Check sheet for the modelled part. Datum: model origin and axes. Units: mm. A direction names the side the tool comes from. Give positions to 0.01 mm unless a question says otherwise; leave off trailing zeros. Order: outer loops, then holes, each group sorted by start corner. A loop starts at its lowest first (then second) coordinate and runs counter-clockwise, first axis right, second up. Notation, with made-up numbers: (34.25, 2.5) -> (57.25, 2.5) arc R30 cw to (57.25, 27.5) -> close; hole circle Ø1 at (4.5, 58). An arc over 180 degrees is marked (long way). One line per question, with ' | ' between items.
```python
from build123d import *

# Parameters (mm, degrees)
BOSS_EXTRUDE1_DEPTH    = 6
SKETCH2_W              = 98
SKETCH2_H              = 80.5
CUT_EXTRUDE1_DEPTH     = 79.33262411
SKETCH5_R              = 1.75
CUT_EXTRUDE4_DEPTH     = 79.33262411
SKETCH6_W              = 8.5
SKETCH6_H              = 20
CUT_EXTRUDE5_DEPTH     = 79.33262411
MOVE_FACE1_OUTLINE_R   = 1.75
MOVE_FACE1_OUTLINE_R_2 = 1.67
MOVE_FACE1_DEPTH       = 6


# Read off the part's stored shape, not the designer's step: Move Face1
with BuildPart() as part:
    # Sketch1 → Boss-Extrude1 (new body)
    with BuildSketch(Plane(origin=(0, 0, 0), x_dir=(1, 0, 0), z_dir=(0, 1, 0))):
        with BuildLine():
            Line((-60, 30), (-60, -30))
            ThreePointArc((-60, -30), (-54.142135624, -44.142135624), (-40, -50))
            Line((-40, -50), (40, -50))
            ThreePointArc((40, -50), (54.142135624, -44.142135624), (60, -30))
            Line((60, -30), (60, 30))
            ThreePointArc((60, 30), (54.142135624, 44.142135624), (40, 50))
            Line((40, 50), (-40, 50))
            ThreePointArc((-40, 50), (-54.142135624, 44.142135624), (-60, 30))
        make_face()
    extrude(amount=BOSS_EXTRUDE1_DEPTH)

    # Sketch2 → Cut-Extrude1 (cut, through all)
    with BuildSketch(Plane(origin=(0, 6, 0), x_dir=(1, 0, 0), z_dir=(0, 1, 0))):
        with Locations((0, -2.25)):
            Rectangle(SKETCH2_W, SKETCH2_H)
    extrude(amount=-CUT_EXTRUDE1_DEPTH, mode=Mode.SUBTRACT)

    # Sketch5 → Cut-Extrude4 (cut, through all)
    with BuildSketch(Plane(origin=(0, 6, 0), x_dir=(1, 0, 0), z_dir=(0, 1, 0))):
        with Locations(Location((53.475, 0, 0), (0, 0, 270))):
            Circle(SKETCH5_R)
        with Locations(Location((-53.709292606, -36.227375296, 0), (0, 0, 270))):
            Circle(SKETCH5_R)
        with Locations(Location((0, 43.45, 0), (0, 0, 270))):
            Circle(SKETCH5_R)
        with Locations(Location((50.558556763, 40.508556763, 0), (0, 0, 270))):
            Circle(SKETCH5_R)
        with Locations(Location((-50.558556763, 40.508556763, 0), (0, 0, 90))):
            Circle(SKETCH5_R)
    extrude(amount=-CUT_EXTRUDE4_DEPTH, mode=Mode.SUBTRACT)

    # Sketch6 → Cut-Extrude5 (cut, through all)
    with BuildSketch(Plane(origin=(0, 6, 0), x_dir=(1, 0, 0), z_dir=(0, 1, 0))):
        with Locations((-53.25, 25)):
            Rectangle(SKETCH6_W, SKETCH6_H)
    extrude(amount=-CUT_EXTRUDE5_DEPTH, mode=Mode.SUBTRACT)

    # Move Face1 outline → Move Face1 (add)
    # profile 1 of 7: a face of its own
    with BuildSketch(Plane(origin=(0, 0, 0), x_dir=(1, 0, 0), z_dir=(0, 1, 0))):
        with BuildLine():
            ThreePointArc((-40, 50.08), (-54.198704166, 44.198704166), (-60.08, 30))
            Line((-60.08, 30), (-60.08, -30))
            ThreePointArc((-60.08, -30), (-54.198704166, -44.198704166), (-40, -50.08))
            Line((-40, -50.08), (40, -50.08))
            ThreePointArc((40, -50.08), (54.198704166, -44.198704166), (60.08, -30))
            Line((60.08, -30), (60.08, 30))
            ThreePointArc((60.08, 30), (54.198704166, 44.198704166), (40, 50.08))
            Line((40, 50.08), (-40, 50.08))
        make_face()
        with BuildLine():
            Line((-60, -30), (-60, 30))
            ThreePointArc((-60, 30), (-54.142135624, 44.142135624), (-40, 50))
            Line((-40, 50), (40, 50))
            ThreePointArc((40, 50), (54.142135624, 44.142135624), (60, 30))
            Line((60, 30), (60, -30))
            ThreePointArc((60, -30), (54.142135624, -44.142135624), (40, -50))
            Line((40, -50), (-40, -50))
            ThreePointArc((-40, -50), (-54.142135624, -44.142135624), (-60, -30))
        make_face(mode=Mode.SUBTRACT)
    # profile 2 of 7: a face of its own
    with BuildSketch(Plane(origin=(0, 0, 0), x_dir=(1, 0, 0), z_dir=(0, 1, 0))):
        Polygon((-57.5, 15), (-49, 15), (-49, -42.5), (49, -42.5), (49, 38), (-49, 38), (-49, 35), (-57.5, 35), align=None)
        Polygon((-48.92, -42.42), (-48.92, 15.08), (-57.42, 15.08), (-57.42, 34.92), (-48.92, 34.92), (-48.92, 37.92), (48.92, 37.92), (48.92, -42.42), align=None, mode=Mode.SUBTRACT)
    # profile 3 of 7: a face of its own
    with BuildSketch(Plane(origin=(0, 0, 0), x_dir=(1, 0, 0), z_dir=(0, 1, 0))):
        with Locations((53.475, 0)):
            Circle(MOVE_FACE1_OUTLINE_R)
        with Locations((53.475, 0)):
            Circle(MOVE_FACE1_OUTLINE_R_2, mode=Mode.SUBTRACT)
    # profile 4 of 7: a face of its own
    with BuildSketch(Plane(origin=(0, 0, 0), x_dir=(1, 0, 0), z_dir=(0, 1, 0))):
        with Locations((0, 43.45)):
            Circle(MOVE_FACE1_OUTLINE_R)
        with Locations((0, 43.45)):
            Circle(MOVE_FACE1_OUTLINE_R_2, mode=Mode.SUBTRACT)
    # profile 5 of 7: a face of its own
    with BuildSketch(Plane(origin=(0, 0, 0), x_dir=(1, 0, 0), z_dir=(0, 1, 0))):
        with Locations((50.558556763, 40.508556763)):
            Circle(MOVE_FACE1_OUTLINE_R)
        with Locations((50.558556763, 40.508556763)):
            Circle(MOVE_FACE1_OUTLINE_R_2, mode=Mode.SUBTRACT)
    # profile 6 of 7: a face of its own
    with BuildSketch(Plane(origin=(0, 0, 0), x_dir=(1, 0, 0), z_dir=(0, 1, 0))):
        with Locations((-50.558556763, 40.508556763)):
            Circle(MOVE_FACE1_OUTLINE_R)
        with Locations((-50.558556763, 40.508556763)):
            Circle(MOVE_FACE1_OUTLINE_R_2, mode=Mode.SUBTRACT)
    # profile 7 of 7: a face of its own
    with BuildSketch(Plane(origin=(0, 0, 0), x_dir=(1, 0, 0), z_dir=(0, 1, 0))):
        with Locations((-53.709292606, -36.227375296)):
            Circle(MOVE_FACE1_OUTLINE_R)
        with Locations((-53.709292606, -36.227375296)):
            Circle(MOVE_FACE1_OUTLINE_R_2, mode=Mode.SUBTRACT)
    extrude(amount=MOVE_FACE1_DEPTH)


solid = part.part
```
Q1. Section check C-C (y = 1.15). Enter the section's corners in (x, z) (3 decimals).
Result sheet:
outline: (-60.08, -30) arc R20.08 ccw to (-40, -50.08) -> (40, -50.08) arc R20.08 ccw to (60.08, -30) -> (60.08, 30) arc R20.08 ccw to (40, 50.08) -> (-40, 50.08) arc R20.08 ccw to (-60.08, 30) -> close; hole (-57.42, -34.92) -> (-48.92, -34.92) -> (-48.92, -37.92) -> (48.92, -37.92) -> (48.92, 42.42) -> (-48.92, 42.42) -> (-48.92, -15.08) -> (-57.42, -15.08) -> close; hole circle Ø3.34 at (-53.709, 36.227); hole circle Ø3.34 at (-50.559, -40.509); hole circle Ø3.34 at (0, -43.45); hole circle Ø3.34 at (50.559, -40.509); hole circle Ø3.34 at (53.475, 0)
Q2. Thickness scan on line 1 (X direction, y = 3.25, z = 0) (3 decimals); line 2 (Z direction, x = 13, y = 2.6); line 3 (X direction, y = 1.5, z = 14.5). Record the ranges inside material, lowest first.
Result sheet:
line 1: x = -60.08 to -48.92, 48.92 to 51.805, 55.145 to 60.08 | line 2: z = -50.08 to -37.92, 42.42 to 50.08 | line 3: x = -60.08 to -48.92, 48.92 to 60.08
Q3. Depth check by flat-ended pin: pin 1 Ø1 at (y, z) = (0.5, 38.5) entering from -X; pin 2 Ø1.8 at (x, y) = (-54, 2) entering from +Z; pin 3 Ø3 at (x, y) = (42.5, 3) entering from +Z; pin 4 Ø4.5 at (x, z) = (0, -43.45) entering from -Y. Enter the tip coordinate at first touch or a pass-through.
Result sheet:
pin 1: stops at x = -58.42 | pin 2: stops at z = 45.22 | pin 3: stops at z = 50.06 | pin 4: stops at y = 0
Q4. Mould release check, pull along X, two halves, no side actions. Record for faces 3 (the face through (54.354, 2.958, -44.042)), 4 (the face through (1, 3, 42.42)), 5 (the face through (-54.354, 2.958, 44.042)): pulls with the +X half, pulls with the -X half, needs draft (parallel to the pull), parting line crosses it, or undercut.
Result sheet:
face 3: pulls with the +X half | face 4: undercut | face 5: pulls with the -X half
Q5. Access from +Z, -Z, +X, -X, +Y, -Y to the whole of each face (thin tool, end or side, straight path). Record for faces 1 (the face through (60.08, 3, 0)), 2 (the face through (-53, 3, -15.08)).
Result sheet:
face 1: +Z, -Z, +X, +Y, -Y | face 2: +Y, -Y
Q6. Section check B-B (z = 5). Enter the section's corners in (x, y).
Result sheet:
outline: (-60.08, 0) -> (-48.92, 0) -> (-48.92, 6) -> (-60.08, 6) -> close; (48.92, 0) -> (60.08, 0) -> (60.08, 6) -> (48.92, 6) -> close
Q7. Section check A-A (x = -11). Enter the section's corners in (y, z), and give its area (3 significant figures).
Result sheet:
outline: (0, -50.08) -> (6, -50.08) -> (6, -37.92) -> (0, -37.92) -> close; (0, 42.42) -> (6, 42.42) -> (6, 50.08) -> (0, 50.08) -> close | area: 119 mm2
